```python
from build123d import *

# Parameters (mm, degrees)
SKETCH_W        = 25
SKETCH_H        = 120
PAD_DEPTH       = 20
SKETCH001_W     = 25
SKETCH001_H     = 4
PAD001_DEPTH    = 10
SKETCH002_R     = 2
POCKET_DEPTH    = 4
SKETCH003_W     = 25
SKETCH003_H     = 4
PAD002_DEPTH    = 10
SKETCH004_R     = 2
POCKET001_DEPTH = 4
SKETCH005_W     = 20.5
SKETCH005_H     = 46
POCKET002_DEPTH = 20


with BuildPart() as part:
    # Sketch → Pad (new body)
    with BuildSketch(Plane.XZ):
        Rectangle(SKETCH_W, SKETCH_H)
    extrude(amount=PAD_DEPTH)

    # Sketch001 → Pad001 (new body)
    with BuildSketch(Plane.XZ.offset(20)):
        with Locations((0, -58)):
            Rectangle(SKETCH001_W, SKETCH001_H)
    extrude(amount=PAD001_DEPTH)

    # Sketch002 → Pocket (cut)
    with BuildSketch(Plane(origin=(0, 0, -60), x_dir=(1, 0, 0), z_dir=(0, 0, -1))):
        with Locations((-6.290528, 24.864162)):
            Circle(SKETCH002_R)
        with Locations((6.061036, 24.804857)):
            Circle(SKETCH002_R)
    extrude(amount=-POCKET_DEPTH, mode=Mode.SUBTRACT)

    # Sketch003 → Pad002 (new body)
    with BuildSketch(Plane(origin=(0, 0, 0), x_dir=(1, 0, 0), z_dir=(0, 1, 0))):
        with Locations((0, 58)):
            Rectangle(SKETCH003_W, SKETCH003_H)
    extrude(amount=PAD002_DEPTH)

    # Sketch004 → Pocket001 (cut)
    with BuildSketch(Plane(origin=(0, 0, -60), x_dir=(1, 0, 0), z_dir=(0, 0, -1))):
        with Locations((-6.25, -5)):
            Circle(SKETCH004_R)
        with Locations((6.25, -5)):
            Circle(SKETCH004_R)
    extrude(amount=-POCKET001_DEPTH, mode=Mode.SUBTRACT)

    # Sketch005 → Pocket002 (cut)
    with BuildSketch(Plane.XZ.offset(20)):
        with Locations((0, 33.891745)):
            Rectangle(SKETCH005_W, SKETCH005_H)
    extrude(amount=-POCKET002_DEPTH, mode=Mode.SUBTRACT)


solid = part.part
```
Input: part model. Units: mm. Frame: model coordinates. A direction names the side the tool comes from. Give positions to 0.01 mm unless a question says otherwise; leave off trailing zeros. Order: outer loops, then holes, each group sorted by start corner. A loop starts at its lowest first (then second) coordinate and runs counter-clockwise, first axis right, second up. Notation, with made-up numbers: M 62.5,16 L 114.5,16 A12 cw 114.5,39 Z; hole C -6.5,-16.75 d9. An arc over 180 degrees is marked long. Return JSON: item names as keys, results as strings.
1) Contact query for flat-ended pins moving along their axis: pin 1 (5 mm diameter, centred on x = -1.5, y = 7.5, fed in from +Z); pin 2 (7.5 mm diameter, centred on x = -1.5, z = 11, fed in from +Y); pin 3 (7.5 mm diameter, centred on x = 1.5, z = 4, fed in from -Y). Output: stop coordinate, or through.
Taken from the geometry:
{"pin 1": "stops at z = -56", "pin 2": "stops at y = 0", "pin 3": "stops at y = -20"}
2) Mould query, pull axis Y, two halves, no side actions, for faces 6 (the face through (0, 10, -58)), 7 (the face through (0, -10, 10.892)), 8 (the face through (-6.551, -26.847, -58.028)). Classes: released by +Y, released by -Y, zero draft, split by the parting line, or undercut.
Taken from the geometry:
{"face 6": "released by +Y", "face 7": "zero draft", "face 8": "undercut"}
3) Section query C-C on y = -18.5. Output: boundary loops of the cut face in (x, z), and give its area (3 significant figures).
Taken from the geometry:
{"outline": "M -12.5,-60 L 12.5,-60 L 12.5,60 L -12.5,60 Z; hole M -10.25,10.89 L 10.25,10.89 L 10.25,56.89 L -10.25,56.89 Z", "area": "2,060 mm2"}
4) Line query: L1, parallel to X at y = 5, z = -58.65; L2, parallel to X at y = -13.5, z = 25; L3, parallel to Z at x = 8.5, y = -13.5. Output: solid intervals per line, ascending. Write a range as [from, to].
Taken from the geometry:
{"L1": "x = [-12.5, -8.25], [-4.25, 4.25], [8.25, 12.5]", "L2": "x = [-12.5, -10.25], [10.25, 12.5]", "L3": "z = [-60, 10.89], [56.89, 60]"}
5) Section query A-A on y = 5. Output: boundary loops of the cut face in (x, z), and give its area (3 significant figures).
Taken from the geometry:
{"outline": "M -12.5,-60 L -8.25,-60 L -8.25,-56 L -12.5,-56 Z; M -4.25,-60 L 4.25,-60 L 4.25,-56 L -4.25,-56 Z; M 8.25,-60 L 12.5,-60 L 12.5,-56 L 8.25,-56 Z", "area": "68.0 mm2"}
6) Section query D-D on x = -6.25. Output: boundary loops of the cut face in (y, z), and give its area (3 significant figures).
Taken from the geometry:
{"outline": "M -30,-60 L -26.86,-60 L -26.86,-56 L -30,-56 Z; M -22.86,-60 L 3,-60 L 3,-56 L 0,-56 L 0,10.89 L -20,10.89 L -20,-56 L -22.86,-56 Z; M -20,56.89 L 0,56.89 L 0,60 L -20,60 Z; M 7,-60 L 10,-60 L 10,-56 L 7,-56 Z", "area": "1,530 mm2"}
7) Section query B-B on x = 2.25. Output: boundary loops of the cut face in (y, z).
Taken from the geometry:
{"outline": "M -30,-60 L 10,-60 L 10,-56 L 0,-56 L 0,10.89 L -20,10.89 L -20,-56 L -30,-56 Z; M -20,56.89 L 0,56.89 L 0,60 L -20,60 Z"}
8) Access query for faces 1 (the face through (0, -10, 56.892)), 2 (the face through (0, -30, -58)), 3 (the face through (0, -25, -56)), 4 (the face through (0, 0, -10)), 5 (the face through (4.663, 6.217, -58.028)). Directions: +Z, -Z, +X, -X, +Y, -Y. A direction counts if a zero-diameter tool reaches every point of the face in a straight line with its end or side. Return the directions, or none.
Taken from the geometry:
{"face 1": "+Y, -Y", "face 2": "+Z, -Z, +X, -X, -Y", "face 3": "+Z, +X, -X, -Y", "face 4": "+Z, +X, -X, +Y", "face 5": "+Z, -Z"}
